Can you work these out from the drawing? Everything is in mm from the part's minimum corner. A direction names the side the tool comes from. Coordinates: 2 decimals unless noted, no trailing zeros. Write each loop counter-clockwise with the first axis right and the second up, starting at its lowest first coordinate (ties: lowest second). Pieces come first, ordered by that corner, then holes. Notation, with made-up numbers: (62, -36) -> (117, -36) arc R22 ccw to (117, -19) -> close; hole circle Ø8 at (-31.75, -27.5). An arc over 180 degrees is marked (long way). Use a Markdown table: item, result. Add a question column.
Item 1: If I drill on line 1 along X through (y, z) = (8, 3.25); line 2 along Z through (x, y) = (13, 5); line 3 along Y through (x, z) = (9.5, 6), over which ranges is the centre line in solid material (lowest first)? Write a range as from..to.
Item 2: Imagine slicing it at C-C, the plane z = 11.75. Write out the boundary of the cut face in (x, y), and give its area (3 significant figures).
Item 3: Imagine slicing it at D-D, the plane y = 3. Write out the boundary of the cut face in (x, z) (3 decimals), and give its area (3 significant figures).
Item 4: Will these pins go through, and if not, where does the flat tip stop? pin 1 Ø0.6 at (y, z) = (11, 13) entering from +X; pin 2 Ø5 at (x, z) = (17.5, 5.5) entering from +Y.
Item 5: If we mould it in two halves opening along Z, with no side actions, what happens to the marked faces 1, 2 and 3? For each: pulls with the +Z half, pulls with the -Z half, needs draft (parallel to the pull), parting line crosses it, or undercut.
Item 6: Imagine slicing it at A-A, the plane x = 18.25. Write out the boundary of the cut face in (y, z).
Item 7: Imagine slicing it at B-B, the plane y = 10.25. Write out the boundary of the cut face in (x, z) (3 decimals), and give its area (3 significant figures).
Item 8: On a 3-axis mill with a long thin cutter (end or side, diameter ignored), from which of +Z, -Z, +X, -X, +Y, -Y can I reach the whole of each face in a straight line? I mean the marked faces 4 and 5. Say none if no direction works.
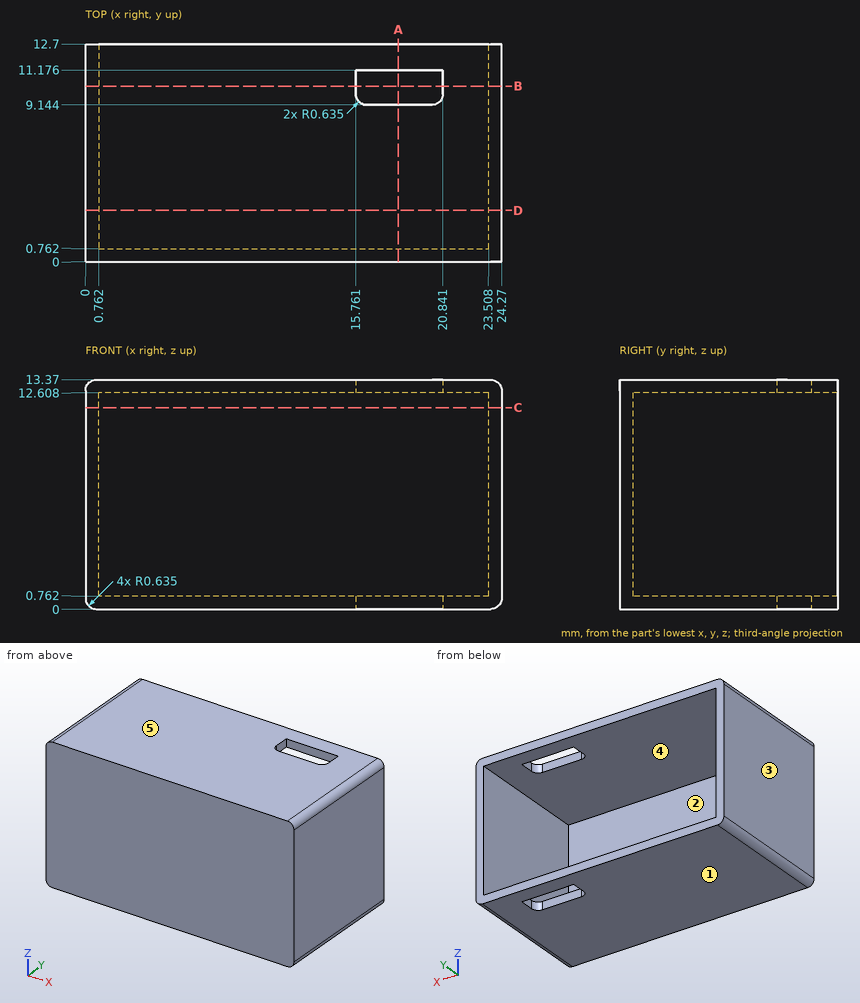
Ans:
| question | item | result |
|---|---|---|
| 1 | line 1 | x = 0..0.76, 23.51..24.27 |
| 1 | line 2 | z = 0..0.76, 12.61..13.37 |
| 1 | line 3 | y = 0..0.76 |
| 2 | outline | (0, 0) -> (24.27, 0) -> (24.27, 12.7) -> (23.51, 12.7) -> (23.51, 0.76) -> (0.76, 0.76) -> (0.76, 12.7) -> (0, 12.7) -> close |
| 2 | area | 36.7 mm^2 |
| 3 | outline | (0, 0.635) arc R0.635 ccw to (0.635, 0) -> (23.635, 0) arc R0.635 ccw to (24.27, 0.635) -> (24.27, 12.735) arc R0.635 ccw to (23.635, 13.37) -> (0.635, 13.37) arc R0.635 ccw to (0, 12.735) -> close; hole (0.762, 0.762) -> (23.508, 0.762) -> (23.508, 12.608) -> (0.762, 12.608) -> close |
| 3 | area | 54.7 mm^2 |
| 4 | pin 1 | stops at x = 24.27 |
| 4 | pin 2 | stops at y = 0.76 |
| 5 | face 1 | pulls with the -Z half |
| 5 | face 2 | undercut |
| 5 | face 3 | needs draft |
| 6 | outline | (0, 0) -> (9.14, 0) -> (9.14, 0.76) -> (0.76, 0.76) -> (0.76, 12.61) -> (9.14, 12.61) -> (9.14, 13.37) -> (0, 13.37) -> close; (11.18, 0) -> (12.7, 0) -> (12.7, 0.76) -> (11.18, 0.76) -> close; (11.18, 12.61) -> (12.7, 12.61) -> (12.7, 13.37) -> (11.18, 13.37) -> close |
| 7 | outline | (0, 0.635) arc R0.635 ccw to (0.635, 0) -> (15.761, 0) -> (15.761, 0.762) -> (0.762, 0.762) -> (0.762, 12.608) -> (15.761, 12.608) -> (15.761, 13.37) -> (0.635, 13.37) arc R0.635 ccw to (0, 12.735) -> close; (20.841, 0) -> (23.635, 0) arc R0.635 ccw to (24.27, 0.635) -> (24.27, 12.735) arc R0.635 ccw to (23.635, 13.37) -> (20.841, 13.37) -> (20.841, 12.608) -> (23.508, 12.608) -> (23.508, 0.762) -> (20.841, 0.762) -> close |
| 7 | area | 47.0 mm^2 |
| 8 | face 4 | +Y |
| 8 | face 5 | +Z, +X, -X, +Y, -Y |
